Could you check a few things on this model? Use its own coordinates, in mm. Round coordinates to 2 decimals unless told otherwise and drop trailing zeros. Loops run counter-clockwise (first coordinate to the right, second up) from the corner with the lowest first, then second, coordinate; pieces in that order, holes last.
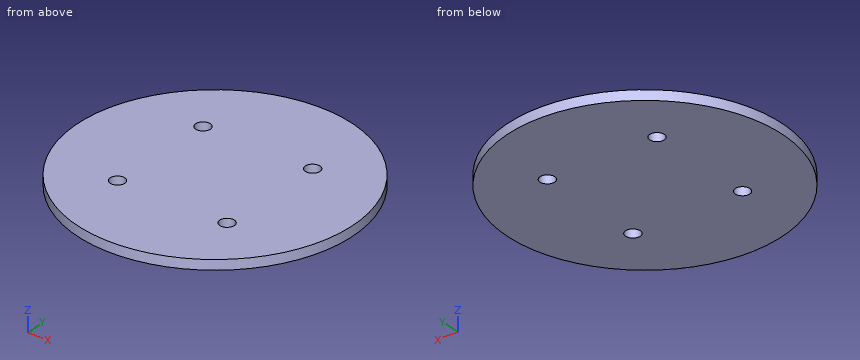
from build123d import *

# Parameters (mm, degrees)
SKETCH1_R               = 88.9
BOSS_EXTRUDE1_DEPTH     = 6.35
CUT_EXTRUDE1_DEPTH      = 126.88384527
CUT_EXTRUDE1_DEPTH_BACK = 126.88384527
SKETCH2_R               = 4.7625


with BuildPart() as part:
    # Sketch1 → Boss-Extrude1 (new body)
    with BuildSketch(Plane.XY):
        Circle(SKETCH1_R)
    extrude(amount=BOSS_EXTRUDE1_DEPTH)

    # Sketch2 → Cut-Extrude1 (cut, two sides: drawn at the far end of the back side and taken through both)
    with BuildSketch(Plane.XY.offset(6.35).offset(-CUT_EXTRUDE1_DEPTH_BACK)):
        with Locations((-35.921024484, 35.921024484)):
            Circle(SKETCH2_R)
        with Locations((35.921024484, 35.921024484)):
            Circle(SKETCH2_R)
        with Locations((35.921024484, -35.921024484)):
            Circle(SKETCH2_R)
        with Locations((-35.921024484, -35.921024484)):
            Circle(SKETCH2_R)
    extrude(amount=CUT_EXTRUDE1_DEPTH + CUT_EXTRUDE1_DEPTH_BACK, mode=Mode.SUBTRACT)


solid = part.part
Item 1: If we section it at A-A, the plane z = 4.75: Please give me the cut outline in (x, y) (1 decimal), then the cut area to 3 significant figures.
Results list:
outline: circle Ø177.8 at (0, 0); hole circle Ø9.5 at (-35.9, -35.9); hole circle Ø9.5 at (-35.9, 35.9); hole circle Ø9.5 at (35.9, -35.9); hole circle Ø9.5 at (35.9, 35.9)
area: 24,500 mm2
Item 2: If we section it at B-B, the plane y = -49: Please give me the cut outline in (x, z).
Results list:
outline: (-74.18, 0) - (74.18, 0) - (74.18, 6.35) - (-74.18, 6.35) - close
Item 3: Will these pins go through, and if not, where does the flat tip stop? pin 1 (2 mm diameter, centred on y = 16.5, z = 2.5, fed in from -X); pin 2 (8.5 mm diameter, centred on x = -35.92, y = 35.92, fed in from +Z).
Results list:
pin 1: stops at x = -87.54
pin 2: passes through
Item 4: If we section it at C-C, the plane x = 16: Please give me the cut outline in (y, z).
Results list:
outline: (-87.45, 0) - (87.45, 0) - (87.45, 6.35) - (-87.45, 6.35) - close
Item 5: If I drill on line 1 along X through (y, z) = (-35, 4.5); line 2 along X through (y, z) = (38.5, 3.5); line 3 along Y through (x, z) = (-33, 2.25), over which ranges is the centre line in solid material (lowest first)?
Results list:
line 1: x = -81.72 to -40.59, -31.25 to 31.25, 40.59 to 81.72
line 2: x = -80.13 to -39.92, -31.92 to 31.92, 39.92 to 80.13
line 3: y = -82.55 to -39.68, -32.16 to 32.16, 39.68 to 82.55
